Check sheet for the drawn part. Datum: minimum x, y, z corner. Units: mm. A direction names the side the tool comes from. Coordinates: 2 decimals unless noted, no trailing zeros. Order: outer loops, then holes, each group sorted by start corner. A loop starts at its lowest first (then second) coordinate and runs counter-clockwise, first axis right, second up. Notation, with made-up numbers: (67.5, 56.25) -> (81.5, 56.25) arc R16 cw to (81.5, 78.25) -> close; hole circle Ø3 at (-20.5, -3). An arc over 180 degrees is marked (long way). Answer as CSV lines item,"result".
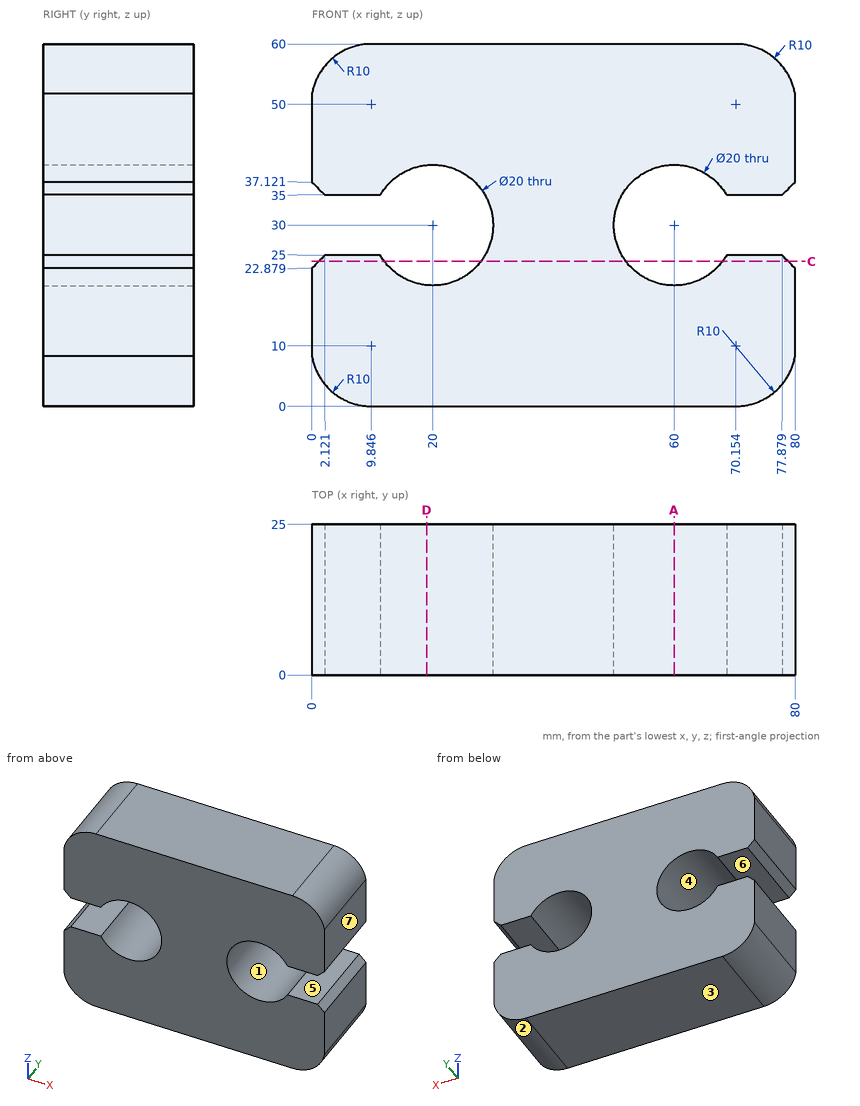
Item 1: Tool access check on the marked faces 5, 6 and 7. Record the directions out of +Z, -Z, +X, -X, +Y, -Y that give a thin tool (end or side, any length) a straight path to the whole face; none if there is none.
Answer list:
face 5,"+X, +Y, -Y"
face 6,"-X, +Y, -Y"
face 7,"+Z, -Z, +X, +Y, -Y"
Item 2: Section check A-A, the plane x = 60. Record the boundary of the cut face in (y, z).
Answer list:
outline,"(0, 0) -> (25, 0) -> (25, 20) -> (0, 20) -> close; (0, 40) -> (25, 40) -> (25, 60) -> (0, 60) -> close"
Item 3: Section check D-D, the plane x = 19. Record the boundary of the cut face in (y, z).
Answer list:
outline,"(0, 0) -> (25, 0) -> (25, 20.05) -> (0, 20.05) -> close; (0, 39.95) -> (25, 39.95) -> (25, 60) -> (0, 60) -> close"
Item 4: Thickness scan on line 1 (Z direction, x = 60, y = 10.25); line 2 (Z direction, x = 12, y = 3.25); line 3 (X direction, y = 10, z = 30). Record the ranges inside material, lowest first.
Answer list:
line 1,"0 to 20, 40 to 60"
line 2,"0 to 24, 36 to 60"
line 3,"30 to 50"
Item 5: Release check for a two-part mould opening along X. For the marked faces 1, 2, 3 and 4 record: +X half, -X half, draft (parallel to the pull), parting line (faces both ways), or undercut.
Answer list:
face 1,"undercut"
face 2,"+X half"
face 3,"draft"
face 4,"undercut"
Item 6: Depth check by flat-ended pin: pin 1 Ø12 at (x, z) = (20, 30) entering from -Y; pin 2 Ø7.5 at (x, y) = (73, 13.5) entering from -Z; pin 3 Ø3 at (x, y) = (5.5, 15) entering from -Z. Enter the tip coordinate at first touch or a pass-through.
Answer list:
pin 1,"through"
pin 2,"z = 0"
pin 3,"z = 0.41"
Item 7: Section check C-C, the plane z = 24. Record the boundary of the cut face in (x, y).
Answer list:
outline,"(1.12, 0) -> (12, 0) -> (12, 25) -> (1.12, 25) -> close; (28, 0) -> (52, 0) -> (52, 25) -> (28, 25) -> close; (68, 0) -> (78.88, 0) -> (78.88, 25) -> (68, 25) -> close"
